```python
from build123d import *

# Parameters (mm, degrees)
EXTRUDE_1_DEPTH = 114
FILLET_5_R      = 2.5
FILLET_6_R      = 2.5
FILLET_8_R      = 2.5
FILLET_10_R     = 2.5
FILLET_11_R     = 2.5


with BuildPart() as part:
    # ｽｹｯﾁ1 → ﾎﾞｽ - 押し出し1 (new body)
    with BuildSketch(Plane(origin=(0, 0, 0), x_dir=(1, 0, 0), z_dir=(0, 1, 0))):
        Polygon((47.807009209, -4.786582838), (36.65910681, -31.7), (5, -31.7), (5, 36.7), (-26, 36.7), (-26, 16.7), (-21, 16.7), (-21, 31.7), (0, 31.7), (0, -36.7), (40, -36.7), (52.426406871, -6.7), align=None)
    extrude(amount=EXTRUDE_1_DEPTH)

    # ﾌｨﾚｯﾄ5
    fillet_5_edges = [part.edges().sort_by_distance(p)[0] for p in [
        (-26, 57, -36.7),
    ]]
    fillet(fillet_5_edges, radius=FILLET_5_R)

    # ﾌｨﾚｯﾄ6
    fillet_6_edges = [part.edges().sort_by_distance(p)[0] for p in [
        (5, 57, -36.7),
    ]]
    fillet(fillet_6_edges, radius=FILLET_6_R)

    # ﾌｨﾚｯﾄ8
    fillet_8_edges = [part.edges().sort_by_distance(p)[0] for p in [
        (52.426406871, 57, 6.7),
        (47.807009209, 57, 4.786582838),
    ]]
    fillet(fillet_8_edges, radius=FILLET_8_R - 0.0001)  # a hair under: the kernel refuses the full size

    # ﾌｨﾚｯﾄ10
    fillet_10_edges = [part.edges().sort_by_distance(p)[0] for p in [
        (0, 57, 36.7),
    ]]
    fillet(fillet_10_edges, radius=FILLET_10_R)

    # ﾌｨﾚｯﾄ11
    fillet_11_edges = [part.edges().sort_by_distance(p)[0] for p in [
        (5, 57, 31.7),
    ]]
    fillet(fillet_11_edges, radius=FILLET_11_R)


solid = part.part
```
Input: part model. Units: mm. Frame: model coordinates. A direction names the side the tool comes from. Give positions to 0.01 mm unless a question says otherwise; leave off trailing zeros. Order: outer loops, then holes, each group sorted by start corner. A loop starts at its lowest first (then second) coordinate and runs counter-clockwise, first axis right, second up. Notation, with made-up numbers: M 84,-3 L 97,-3 A11 cw 97,14 Z; hole C -2,-32 d6. An arc over 180 degrees is marked long. One line per question, with ' | ' between items. Start each with the question number.
1. Section query C-C (z = 12.5). Return the cut outline in (x, y), and give its area (3 significant figures).
2. First-contact query: pin 1 Ø19 at (y, z) = (42.5, -12.5) entering from +X; pin 2 Ø5.5 at (x, y) = (-22.5, 58.5) entering from +Z; pin 3 Ø6 at (x, z) = (1, 11.5) entering from -Y; pin 4 Ø6.5 at (x, y) = (-11, 59) entering from +Z. Flat tips, straight axial feed; report the tip coordinate or a pass-through.
3. Section query A-A (z = -19.5). Return the cut outline in (x, y), and give its area (3 significant figures).
4. Material intervals for probe 1 along X at (y, z) = (103, -28); probe 2 along Z at (x, y) = (13, 51.5); probe 3 along X at (y, z) = (23.5, -4), sorted ascending. Write a range as [from, to].
5. Pull-direction query (X, two-part tool) for faces 6 (the face through (5.752, 57.798, 30.987)), 7 (the face through (-21, 56, -24)), 8 (the face through (51.46, 57.8, 7.07)), 9 (the face through (-10, 56, -36.7)); classes: released by +X, released by -X, zero draft, split by the parting line, or undercut.
6. Section query D-D (x = 11). Return the cut outline in (y, z).
7. Access query for faces 1 (the face through (4, 114, 3)), 2 (the face through (-11, 56, -31.7)), 3 (the face through (22, 56, 31.7)), 4 (the face through (-24, 56, -16.7)), 5 (the face through (4.248, 57.798, -35.987)). Directions: +Z, -Z, +X, -X, +Y, -Y. A direction counts if a zero-diameter tool reaches every point of the face in a straight line with its end or side. Return the directions, or none.
Here are the results:
1) outline: M 0,0 L 5,0 L 5,114 L 0,114 Z; M 44.61,0 L 50.02,0 L 50.02,114 L 44.61,114 Z | area: 1,190 mm²
2) pin 1: x = 5 | pin 2: z = -16.7 | pin 3: y = 0 | pin 4: z = -31.7
3) outline: M -26,0 L -21,0 L -21,114 L -26,114 Z; M 0,0 L 5,0 L 5,114 L 0,114 Z | area: 1,140 mm²
4) probe 1: [-26, -21], [0, 5] | probe 2: [31.7, 36.7] | probe 3: [0, 5]
5) face 6: undercut | face 7: undercut | face 8: released by +X | face 9: zero draft
6) outline: M 0,31.7 L 114,31.7 L 114,36.7 L 0,36.7 Z
7) face 1: +Z, -Z, +X, -X, +Y | face 2: +Z, +Y, -Y | face 3: -Z, +Y, -Y | face 4: +Z, -X, +Y, -Y | face 5: -Z, +X, +Y, -Y
